Read the model definition and answer for the solid it produces. Units are mm, in the model's axes. Face numbers are marked on the shaded views. Give positions to 0.01 mm unless a question says otherwise; leave off trailing zeros. Loops run counter-clockwise (first coordinate to the right, second up) from the corner with the lowest first, then second, coordinate; pieces in that order, holes last. Notation, with made-up numbers: (-11.75, 6.5) - (23.25, 6.5) arc R28 ccw to (23.25, 24.5) - close; hole circle Ø4 at (52.5, 49.5). An arc over 180 degrees is marked (long way). Use a Markdown table: item, result. Add a question column.
Item 1: Each of these flat-tipped pins is pushed along its axis until it touches: P1, Ø0.6, axis at x = 4.5, z = 1, coming from the -Y side; P2, Ø1, axis at y = 14.5, z = 1.5, coming from the +X side; P3, Ø1, axis at y = 10, z = 1, coming from the +X side. Where does it stop, or does it pass through?
Item 2: A cutting plane is placed at A-A (y = 8.5). Give the number of separate pieces and of enclosed holes in the cut face, plus the area to 3 significant figures.
Item 3: A cutting plane is placed at B-B (x = 29.5). Determine the outline of the cut face in (y, z).
Item 4: For a pull along Z with two mould halves and no side action, classify the marked faces 1 and 2 as +Z half, -Z half, draft (parallel to the pull), parting line (faces both ways), or undercut.
Item 5: Consider probe 1 along X at (y, z) = (23, 0.6); probe 2 along Y at (x, z) = (-39, 1.1); probe 3 along Y at (x, z) = (-6, 1.6). Determine where each line is inside the solid, lowest interval first. Write a range as [from, to].
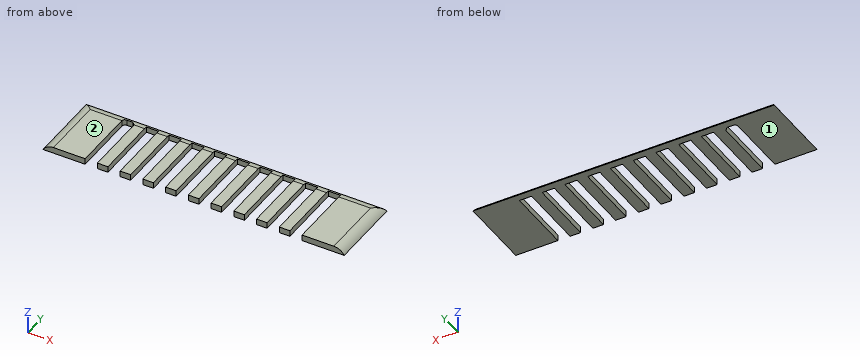
from build123d import *

# Parameters (mm, degrees)
F1_DEPTH    = 2
F2_T1_DEPTH = 67.3205080757
F3_T1_DEPTH = 38.2564064606
F5_R        = 1
F6_SIZE     = 1


# Not quite as in the source:
# - a fillet or chamfer that OpenCascade refuses, or shapes differently, is made with other operations: its cross-section is extruded or revolved along the edge and cut away or added


with BuildPart() as f1:
    # F0 (on Top) → F1 (new body)
    with BuildSketch(Plane.XY):
        Polygon((-1.75, 0), (0, 0), (0, 24.4), (-50, 24.4), (-50, 0), (-36, 0), (-36, 22), (-31.95, 22), (-31.95, 0), (-28.45, 0), (-28.45, 22), (-24.4, 22), (-24.4, 0), (-20.9, 0), (-20.9, 22), (-16.85, 22), (-16.85, 0), (-13.35, 0), (-13.35, 22), (-9.3, 22), (-9.3, 0), (-5.8, 0), (-5.8, 22), (-1.75, 22), align=None)
    extrude(amount=F1_DEPTH)

    # F2: fillet of radius 4 on 1 edges, made by hand

    # F2_s2 → F2_t1 (cut)
    with BuildSketch(Plane.YZ.offset(-58.6602540378)):
        with BuildLine():
            ThreePointArc((24.4, 0), (22.9358983849, 1.4641016151), (20.9358983849, 2))
            Line((20.9358983849, 2), (24.4, 2))
            Line((24.4, 2), (24.4, 0))
        make_face()
    extrude(amount=F2_T1_DEPTH, mode=Mode.SUBTRACT)

    # F3: fillet of radius 4 on 1 edges, made by hand

    # F3_s2 → F3_t1 (cut)
    with BuildSketch(Plane.XZ.offset(-29.5961524227)):
        with BuildLine():
            ThreePointArc((-50, 0), (-48.5358983849, 1.4641016151), (-46.5358983849, 2))
            Line((-46.5358983849, 2), (-50, 2))
            Line((-50, 2), (-50, 0))
        make_face()
    extrude(amount=F3_T1_DEPTH, mode=Mode.SUBTRACT)

    # F4: F1 across plane


with BuildPart() as f1_1:
    add(f1.part)
    add(f1.part.mirror(Plane.YZ))

    # F5
    f5_edges = [f1_1.edges().sort_by_distance(p)[0] for p in [
        (-36, 22, 0.927932),
    ]]
    fillet(f5_edges, radius=F5_R)

    # F6
    f6_edges = [f1_1.edges().sort_by_distance(p)[0] for p in [
        (-31.95, 22, 0.927932),
    ]]
    chamfer(f6_edges, length=F6_SIZE)


solid = f1_1.part
Geometry says:
| question | item | result |
|---|---|---|
| 1 | P1 | y = 22 |
| 1 | P2 | x = 49.18 |
| 1 | P3 | x = 49.66 |
| 2 | separate pieces | 11 |
| 2 | enclosed holes | 0 |
| 2 | area | 115 mm² |
| 3 | outline | (0, 0) - (24.4, 0) arc R4 ccw to (20.94, 2) - (0, 2) - close |
| 4 | face 1 | -Z half |
| 4 | face 2 | +Z half |
| 5 | probe 1 | [-49.58, 49.58] |
| 5 | probe 2 | [0, 23.46] |
| 5 | probe 3 | [0, 22.68] |
